Source: CAD feature listing. Evaluate the final solid. Frame: model axes, mm. Face numbers are marked on the shaded views. A direction names the side the tool comes from. Coordinates: 2 decimals unless noted, no trailing zeros. Write each loop counter-clockwise with the first axis right and the second up, starting at its lowest first coordinate (ties: lowest second). Pieces come first, ordered by that corner, then holes. Notation, with made-up numbers: M 8.25,7 L 60.25,7 A13 ccw 60.25,26 Z; hole C 26.5,2 d1. An arc over 180 degrees is marked long. Write item = value, one per line. Start each with the question number.
1. Pin query (flat end, axial travel): pin 1 Ø2 at (x, y) = (-4, -1.5) entering from -Z. Return the tip coordinate at first contact, or that it passes through.
2. Section query B-B (y = 0). Output: boundary loops of the cut face in (x, z).
3. Pull-direction query (Y, two-part tool) for the marked faces 1, 2 and 3; classes: pulls with the +Y half, pulls with the -Y half, needs draft (parallel to the pull), parting line crosses it, or undercut.
4. Line query: line 1 along X through (y, z) = (-0.3, -0.8); line 2 along Z through (x, y) = (-3.55, 0.4); line 3 along Y through (x, z) = (-3.1, 1.05). Output: solid intervals per line, ascending.
5. Section query C-C (x = -0.55). Output: boundary loops of the cut face in (y, z).
6. Access query for the marked faces 4 and 5. Directions: +Z, -Z, +X, -X, +Y, -Y. A direction counts if a zero-diameter tool reaches every point of the face in a straight line with its end or side. Return the directions, or none.
7. Section query A-A (x = -4.1). Output: boundary loops of the cut face in (y, z), then the cut area to 3 significant figures.
```python
from build123d import *

# Parameters (mm, degrees)
CUT_EXTRUDE1_DEPTH = 2


with BuildPart() as part:
    # Sketch1 → Revolve1 (revolve)
    with BuildSketch(Plane.XY, mode=Mode.PRIVATE) as revolve1_sk:
        Polygon((0, 0), (0, 1.75), (-0.75, 2.5), (-4.717098368, 2.5), (-5, 2.01), (-5, 0), align=None)
    revolve(revolve1_sk.sketch.rotate(Axis((-5, 0, 0), (1, 0, 0)), 90), axis=Axis((-5, 0, 0), (1, 0, 0)))

    # Sketch2 → Cut-Extrude1 (cut)
    with BuildSketch(Plane(origin=(-5, 0, 0), x_dir=(0, 0, -1), z_dir=(1, 0, 0))):
        Polygon((1.25, -0.721687836), (1.25, 0.721687836), (0, 1.443375673), (-1.25, 0.721687836), (-1.25, -0.721687836), (0, -1.443375673), align=None)
    extrude(amount=CUT_EXTRUDE1_DEPTH, mode=Mode.SUBTRACT)


solid = part.part
```
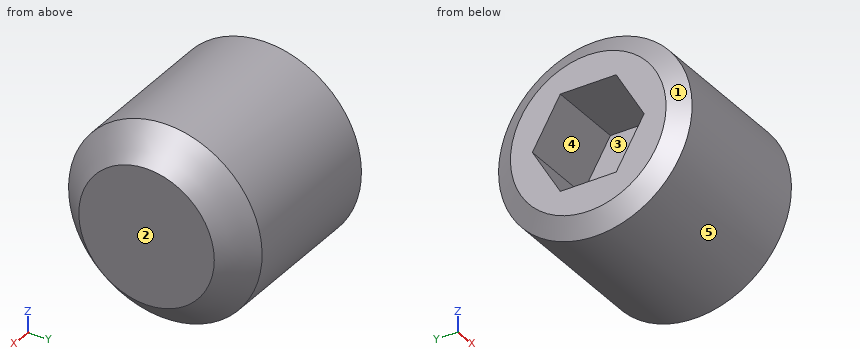
Results are:
q1.pin_1 = -2.45
q2.outline = M -5,-2.01 L -4.72,-2.5 L -0.75,-2.5 L 0,-1.75 L 0,1.75 L -0.75,2.5 L -4.72,2.5 L -5,2.01 L -5,1.25 L -3,1.25 L -3,-1.25 L -5,-1.25 Z
q3.face_1 = parting line crosses it
q3.face_2 = needs draft
q3.face_3 = undercut
q4.line_1 = -3 to 0
q4.line_2 = -2.47 to -1.25, 1.25 to 2.47
q4.line_3 = -2.27 to -0.84, 0.84 to 2.27
q5.outline = C 0,0 d4.6
q6.face_4 = -X
q6.face_5 = +X, -X
q7.outline = C 0,0 d5; hole M -1.44,0 L -0.72,-1.25 L 0.72,-1.25 L 1.44,0 L 0.72,1.25 L -0.72,1.25 Z
q7.area = 14.2 mm^2
